Design review of the part shown in the three views and the two pictorial views. Dimensions are in mm from the part's minimum x, y and z. A direction names the side the tool comes from. Give positions to 0.01 mm unless a question says otherwise; leave off trailing zeros. Loops run counter-clockwise (first coordinate to the right, second up) from the corner with the lowest first, then second, coordinate; pieces in that order, holes last. Notation, with made-up numbers: (57.25, 60.25) - (69.25, 60.25) arc R20 ccw to (69.25, 76.25) - close; hole circle Ø7 at (-39, -12.75). An arc over 180 degrees is marked (long way). Answer in a Markdown table with one row per item.
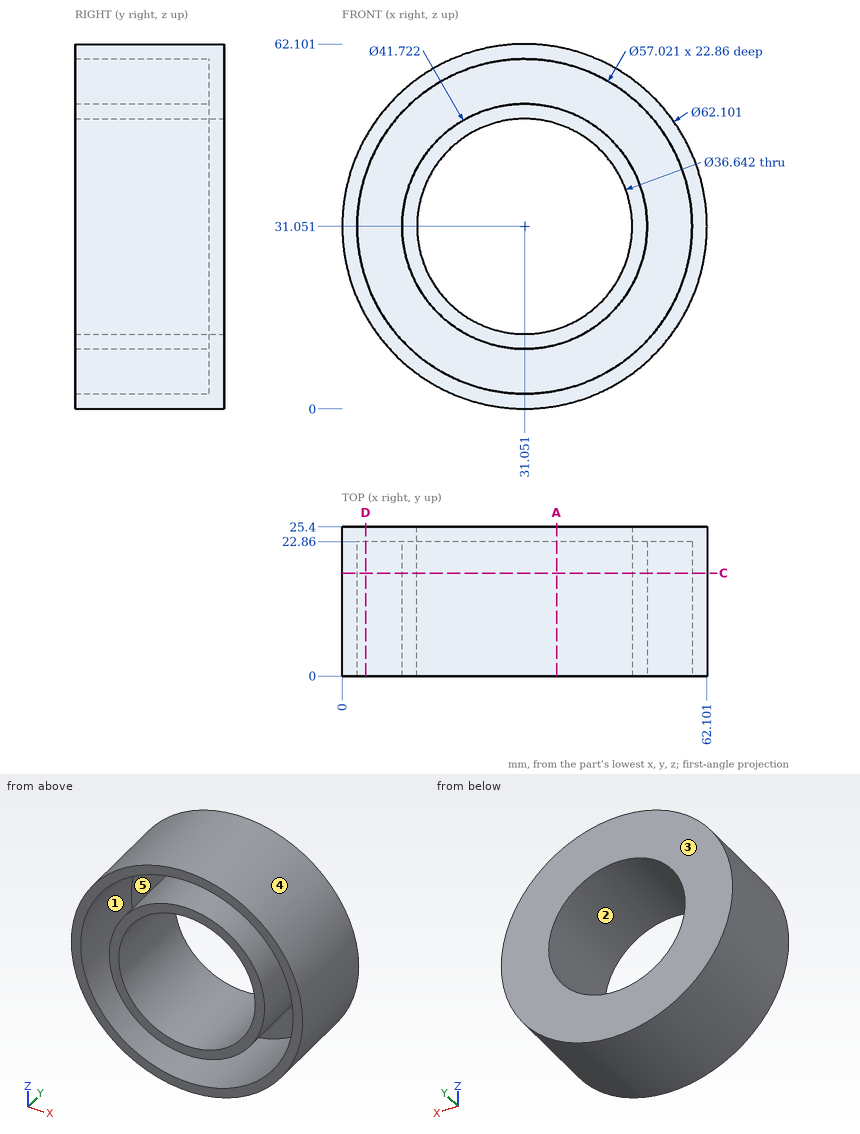
1. For the marked faces 1 and 2, list the 3-axis set-ups (+Z, -Z, +X, -X, +Y, -Y) from which the entire face can be reached by the end or side of a thin tool; tool diameter is ignored.
Values:
| item | result |
|---|---|
| face 1 | -Y |
| face 2 | +Y, -Y |
2. Wall thickness on line 1 (X direction, y = 19.5, z = 16) (1 decimal); line 2 (Z direction, x = 17.5, y = 2) (1 decimal); line 3 (X direction, y = 3.5, z = 41.5) (1 decimal): over which ranges is each line inside the solid? List them lowest first. Write a range as [from, to].
Values:
| item | result |
|---|---|
| line 1 | x = [3.9, 6.8], [16.6, 20.6], [41.5, 45.5], [55.3, 58.2] |
| line 2 | z = [3.1, 6], [15.2, 18.7], [43.4, 46.9], [56.1, 59] |
| line 3 | x = [1.8, 4.5], [13, 16], [46.1, 49.1], [57.6, 60.3] |
3. Clearance check with flat-ended pins moving along their axes: pin 1 (1 mm diameter, centred on x = 51, y = 22, fed in from -Z) (1 decimal); pin 2 (5 mm diameter, centred on y = 11, z = 21.5, fed in from +X); pin 3 (1.5 mm diameter, centred on y = 19, z = 7, fed in from +X) (1 decimal). State where each tip first meets the part, or that it passes through.
Values:
| item | result |
|---|---|
| pin 1 | stops at z = 6.8 |
| pin 2 | stops at x = 61.29 |
| pin 3 | stops at x = 51.6 |
4. We need section C-C, the plane y = 17.5. Give the boundary of the cut face in (x, z).
Values:
| item | result |
|---|---|
| outline | circle Ø62.1 at (31.05, 31.05); circle Ø41.72 at (31.05, 31.05); hole circle Ø57.02 at (31.05, 31.05); hole circle Ø36.64 at (31.05, 31.05) |
5. We need section D-D, the plane x = 4. Give the boundary of the cut face in (y, z) (1 decimal).
Values:
| item | result |
|---|---|
| outline | (0, 15.8) - (25.4, 15.8) - (25.4, 46.3) - (0, 46.3) - (0, 40.1) - (22.9, 40.1) - (22.9, 22) - (0, 22) - close |
6. Mouldability with a two-part tool opening along X and no side actions: class the marked faces 3, 4 and 5 as released by +X, released by -X, zero draft, split by the parting line, or undercut.
Values:
| item | result |
|---|---|
| face 3 | zero draft |
| face 4 | split by the parting line |
| face 5 | undercut |
7. We need section A-A, the plane x = 36.5. Give the boundary of the cut face in (y, z) (1 decimal).
Values:
| item | result |
|---|---|
| outline | (0, 0.5) - (25.4, 0.5) - (25.4, 13.6) - (0, 13.6) - (0, 10.9) - (22.9, 10.9) - (22.9, 3.1) - (0, 3.1) - close; (0, 48.5) - (25.4, 48.5) - (25.4, 61.6) - (0, 61.6) - (0, 59) - (22.9, 59) - (22.9, 51.2) - (0, 51.2) - close |
